from build123d import *

# Parameters (mm, degrees)
EXTRUDE_1_DEPTH     = 160
CUT_EXTRUDE_1_REACH = 164.072
SKETCH_2_R          = 1.95
FILLET_1_R          = 2


with BuildPart() as part:
    # 草图1 → 凸台-拉伸1 (new body)
    with BuildSketch(Plane.XY):
        Polygon((0, 0), (0, 6.5), (25, 6.5), (25, 3.5), (15, 3.5), (15, 0), align=None)
    extrude(amount=EXTRUDE_1_DEPTH)

    # 草图2 → 切除-拉伸1 (cut, up to next)
    with BuildSketch(Plane.XZ, mode=Mode.PRIVATE) as cut_extrude_1_sk1:
        with Locations(Location((7.5, 140, 0), (0, 0, 270))):
            Circle(SKETCH_2_R)
    cut_extrude_1_tool1 = extrude(cut_extrude_1_sk1.sketch, amount=-CUT_EXTRUDE_1_REACH, mode=Mode.PRIVATE) & part.part
    # 草图2 → 切除-拉伸1 (cut, up to next)
    with BuildSketch(Plane.XZ, mode=Mode.PRIVATE) as cut_extrude_1_sk2:
        with Locations(Location((7.5, 20, 0), (0, 0, 270))):
            Circle(SKETCH_2_R)
    cut_extrude_1_tool2 = extrude(cut_extrude_1_sk2.sketch, amount=-CUT_EXTRUDE_1_REACH, mode=Mode.PRIVATE) & part.part
    add(cut_extrude_1_tool1.solids().sort_by_distance((7.5, 0, 140))[0], mode=Mode.SUBTRACT)
    add(cut_extrude_1_tool2.solids().sort_by_distance((7.5, 0, 20))[0], mode=Mode.SUBTRACT)

    # 圆角1
    fillet_1_edges = [part.edges().sort_by_distance(p)[0] for p in [
        (25, 5, 160),
        (0, 3.25, 160),
        (0, 3.25, 0),
        (25, 5, 0),
        (15, 1.75, 0),
        (15, 1.75, 160),
    ]]
    fillet(fillet_1_edges, radius=FILLET_1_R)


solid = part.part
Input: part model. Units: mm. Frame: model coordinates. A direction names the side the tool comes from. Coordinates: 2 decimals unless noted, no trailing zeros. Order: outer loops, then holes, each group sorted by start corner. A loop starts at its lowest first (then second) coordinate and runs counter-clockwise, first axis right, second up. Notation, with made-up numbers: M -25.5,74.5 L 25.5,74.5 A19 ccw 25.5,105.5 Z; hole C 77.25,55.5 d10. An arc over 180 degrees is marked long. Answer in a Markdown table with one row per item.
(1) Access query for faces 1 (the flat face through (8, 0, 79)), 2 (the flat face through (15, 2, 79)). Directions: +Z, -Z, +X, -X, +Y, -Y. A direction counts if a zero-diameter tool reaches every point of the face in a straight line with its end or side. Return the directions, or none.
Numbers:
| item | result |
|---|---|
| face 1 | +Z, -Z, +X, -X, -Y |
| face 2 | +Z, -Z, +X, -Y |
(2) Contact query for flat-ended pins moving along their axis: pin 1 Ø3 at (y, z) = (1.5, 70.5) entering from +X; pin 2 Ø3.5 at (x, z) = (17, 43) entering from -Y. Output: stop coordinate, or through.
Numbers:
| item | result |
|---|---|
| pin 1 | stops at x = 15 |
| pin 2 | stops at y = 3.5 |
(3) Section query A-A, the plane x = 7.5. Output: boundary loops of the cut face in (y, z), plus the area to 3 significant figures.
Numbers:
| item | result |
|---|---|
| outline | M 0,0 L 6.5,0 L 6.5,18.05 L 0,18.05 Z; M 0,21.95 L 6.5,21.95 L 6.5,138.05 L 0,138.05 Z; M 0,141.95 L 6.5,141.95 L 6.5,160 L 0,160 Z |
| area | 989 mm^2 |
(4) Draft query along Z for faces 3 (the cylindrical face through (7.586, 3.204, 21.948)), 4 (the cylindrical face through (8.09, 3.2, 138.14)), 5 (the flat face through (10, 4, 0)), 6 (the flat face through (0, 3, 79)). Return one class per face: pulls with the +Z half, pulls with the -Z half, needs draft (parallel to the pull), parting line crosses it, or undercut.
Numbers:
| item | result |
|---|---|
| face 3 | undercut |
| face 4 | undercut |
| face 5 | pulls with the -Z half |
| face 6 | needs draft |
(5) Material intervals for line 1 (X direction, y = 4.25, z = 20); line 2 (X direction, y = 3.25, z = 20); line 3 (Y direction, x = 18, z = 110.5), sorted ascending. Write a range as [from, to].
Numbers:
| item | result |
|---|---|
| line 1 | x = [0, 5.55], [9.45, 25] |
| line 2 | x = [0, 5.55], [9.45, 15] |
| line 3 | y = [3.5, 6.5] |
(6) Section query C-C, the plane z = 140. Output: boundary loops of the cut face in (x, y), plus the area to 3 significant figures.
Numbers:
| item | result |
|---|---|
| outline | M 0,0 L 5.55,0 L 5.55,6.5 L 0,6.5 Z; M 9.45,0 L 15,0 L 15,3.5 L 25,3.5 L 25,6.5 L 9.45,6.5 Z |
| area | 102 mm^2 |
(7) Section query D-D, the plane z = 10. Output: boundary loops of the cut face in (x, y).
Numbers:
| item | result |
|---|---|
| outline | M 0,0 L 15,0 L 15,3.5 L 25,3.5 L 25,6.5 L 0,6.5 Z |
(8) Section query B-B, the plane y = 2.25. Output: boundary loops of the cut face in (x, z).
Numbers:
| item | result |
|---|---|
| outline | M 0,2 A2 ccw 2,0 L 13,0 A2 ccw 15,2 L 15,158 A2 ccw 13,160 L 2,160 A2 ccw 0,158 Z; hole C 7.5,20 d3.9; hole C 7.5,140 d3.9 |
